```python
from build123d import *

# Parameters (mm, degrees)
SKETCH1_R           = 5.7785
BOSS_EXTRUDE1_DEPTH = 25.4
CUT_EXTRUDE1_REACH  = 40.853
SKETCH2_R           = 2.54
SKETCH3_W           = 5.969
SKETCH3_H           = 4.005387026
CUT_EXTRUDE2_DEPTH  = 33.988295999
FILLET1_R           = 1.27
CUT_EXTRUDE4_DEPTH  = 31.887708266


with BuildPart() as part:
    # Sketch1 → Boss-Extrude1 (new body)
    with BuildSketch(Plane(origin=(0, 0, 0), x_dir=(0, 0, -1), z_dir=(1, 0, 0))):
        with BuildLine():
            Line((-8.9535, 19.05), (-8.9535, 0))
            ThreePointArc((-8.9535, 0), (0, -8.9535), (8.9535, 0))
            Line((8.9535, 0), (8.9535, 19.05))
            Line((8.9535, 19.05), (-8.9535, 19.05))
        make_face()
        Circle(SKETCH1_R, mode=Mode.SUBTRACT)
    extrude(amount=BOSS_EXTRUDE1_DEPTH)

    # Sketch2 → Cut-Extrude1 (cut, up to next)
    with BuildSketch(Plane(origin=(0, 19.05, 0), x_dir=(1, 0, 0), z_dir=(0, 1, 0)), mode=Mode.PRIVATE) as cut_extrude1_sk1:
        with Locations(Location((12.7, 0, 0), (0, 0, 270))):
            Circle(SKETCH2_R)
    cut_extrude1_tool1 = extrude(cut_extrude1_sk1.sketch, amount=-CUT_EXTRUDE1_REACH, mode=Mode.PRIVATE) & part.part
    add(cut_extrude1_tool1.solids().sort_by_distance((12.7, 19.05, 0))[0], mode=Mode.SUBTRACT)
    add(cut_extrude1_tool1.solids().sort_by_distance((12.7, 19.05, 0))[1], mode=Mode.SUBTRACT)

    # Sketch3 → Cut-Extrude2 (cut, through all)
    with BuildSketch(Plane.ZY):
        with Locations((0, -6.950806487)):
            Rectangle(SKETCH3_W, SKETCH3_H)
    extrude(amount=-CUT_EXTRUDE2_DEPTH, mode=Mode.SUBTRACT)

    # Fillet1
    fillet1_edges = [part.edges().sort_by_distance(p)[0] for p in [
        (0, 5.031748975, 2.84122588),
        (0, -6.694776864, 2.9845),
        (25.4, 5.031748975, 2.84122588),
        (0, -6.694776864, -2.9845),
        (25.4, -6.694776864, -2.9845),
        (25.4, -6.694776864, 2.9845),
    ]]
    fillet(fillet1_edges, radius=FILLET1_R)

    # Sketch6 → Cut-Extrude4 (cut, through all)
    with BuildSketch(Plane(origin=(16.4465, 0, -8.9535), x_dir=(1, 0, 0), z_dir=(0, 0, 1))):
        with BuildLine():
            Line((5.6515, 14.282208418), (-3.7465, 14.282208418))
            ThreePointArc((-3.7465, 14.282208418), (-4.5085, 13.520208418), (-3.7465, 12.758208418))
            Line((-3.7465, 12.758208418), (5.6515, 12.758208418))
            Line((5.6515, 12.758208418), (5.6515, 14.282208418))
        make_face()
    extrude(amount=CUT_EXTRUDE4_DEPTH, mode=Mode.SUBTRACT)


solid = part.part
```
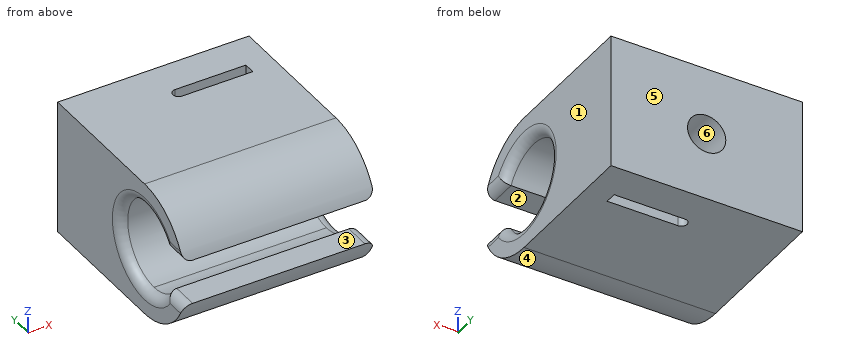
Verification items for the finished model (mm, model axes). Face numbers are marked on the shaded views. A direction names the side the tool comes from. Round coordinates to 2 decimals unless told otherwise and drop trailing zeros. Order: outer loops, then holes, each group sorted by start corner. A loop starts at its lowest first (then second) coordinate and runs counter-clockwise, first axis right, second up. Notation, with made-up numbers: (86.25, -26.5) -> (135.25, -26.5) arc R19 ccw to (135.25, -0.5) -> close; hole circle Ø2 at (5, 23). An arc over 180 degrees is marked (long way). Put each result on its own line as item: value. Start each with the question number.
(1) Section check C-C (y = 14.75). Enter the section's corners in (x, z), then the cut area to 3 significant figures.
(2) Draft check along Z on the marked faces 3, 4, 5 and 6. Enter one of: +Z half, -Z half, draft (parallel to the pull), parting line (faces both ways), or undercut.
(3) Section check B-B (z = 0). Enter the section's corners in (x, y), then the cut area to 3 significant figures.
(4) Tool access check on the marked faces 1 and 2. Record the directions out of +Z, -Z, +X, -X, +Y, -Y that give a thin tool (end or side, any length) a straight path to the whole face; none if there is none.
(5) Material ranges on line 1 along Y through (x, z) = (16.25, -3.5); line 2 along Z through (x, y) = (12.7, 12.25); line 3 along Y through (x, z) = (10.75, -4.5), recorded low to high.
(6) Section check A-A (x = 17). Enter the section's corners in (y, z), then the cut area to 3 significant figures.
(7) Section check D-D (x = 1.75). Enter the section's corners in (y, z).
(8) Depth check by flat-ended pin: pin 1 Ø5 at (x, y) = (11, -3) entering from -Z; pin 2 Ø0.5 at (y, z) = (13.5, -4) entering from -X; pin 3 Ø5 at (x, y) = (15, -4.5) entering from +Z; pin 4 Ø8 at (x, z) = (16.5, -5) entering from -Y. Enter the tip coordinate at first touch or a pass-through.
Completed:
1. outline: (0, -8.95) -> (25.4, -8.95) -> (25.4, 8.95) -> (0, 8.95) -> close; hole circle Ø5.08 at (12.7, 0)
1. area: 435 mm2
2. face 3: undercut
2. face 4: -Z half
2. face 5: draft
2. face 6: undercut
3. outline: (0, 7.05) arc R1.27 ccw to (1.27, 5.78) -> (10.16, 5.78) -> (10.16, 19.05) -> (0, 19.05) -> close; (15.24, 5.78) -> (24.13, 5.78) arc R1.27 ccw to (25.4, 7.05) -> (25.4, 19.05) -> (15.24, 19.05) -> (15.24, 14.28) -> (22.1, 14.28) -> (22.1, 12.76) -> (15.24, 12.76) -> close
3. area: 259 mm2
4. face 1: +Z, -Z, +X, +Y, -Y
4. face 2: +X, -X, -Y
5. line 1: y = -8.24 to -4.6, 4.6 to 12.76, 14.28 to 19.05
5. line 2: z = -8.95 to -2.54, 2.54 to 8.95
5. line 3: y = -7.74 to -3.63, 3.63 to 19.05
6. outline: (-8.44, -2.98) arc R8.95 ccw to (0, -8.95) -> (12.76, -8.95) -> (12.76, 8.95) -> (0, 8.95) arc R8.95 ccw to (-8.44, 2.98) -> (-4.95, 2.98) arc R5.78 cw (long way) to (-4.95, -2.98) -> close; (14.28, -8.95) -> (19.05, -8.95) -> (19.05, 8.95) -> (14.28, 8.95) -> close
6. area: 315 mm2
7. outline: (-8.44, -2.98) arc R8.95 ccw to (0, -8.95) -> (19.05, -8.95) -> (19.05, 8.95) -> (0, 8.95) arc R8.95 ccw to (-8.44, 2.98) -> (-4.95, 2.98) arc R5.78 cw (long way) to (-4.95, -2.98) -> close
8. pin 1: stops at z = -8.94
8. pin 2: stops at x = 0
8. pin 3: stops at z = 8.73
8. pin 4: stops at y = -8.44
